Can you work these out from the model? Positions are in its coordinate system, mm. Round coordinates to 2 decimals unless told otherwise and drop trailing zeros. Loops run counter-clockwise (first coordinate to the right, second up) from the corner with the lowest first, then second, coordinate; pieces in that order, holes last.
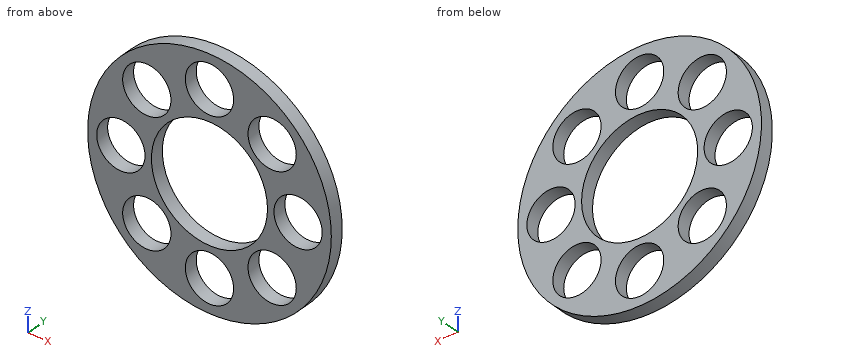
from build123d import *

# Parameters (mm, degrees)
F0_R     = 106
F0_R_2   = 50.5
F1_DEPTH = 6
F2_R     = 21
F3_DEPTH = 12
F4_DEPTH = 25


with BuildPart() as f1:
    # F0 (on Front) → F1 (new body, symmetric)
    with BuildSketch(Plane.XZ):
        Circle(F0_R)
        Circle(F0_R_2, mode=Mode.SUBTRACT)
    extrude(amount=F1_DEPTH, both=True)

    # F2 (on face) → F3 (join)
    with BuildSketch(Plane.XZ.offset(6)):
        with Locations((0, 77.0860096719)):
            Circle(F2_R)
        with Locations((54.5080401736, 54.5080401736)):
            Circle(F2_R)
        with Locations((77.0860096719, 0)):
            Circle(F2_R)
        with Locations((54.5080401736, -54.5080401736)):
            Circle(F2_R)
        with Locations((0, -77.0860096719)):
            Circle(F2_R)
        with Locations((-54.5080401736, -54.5080401736)):
            Circle(F2_R)
        with Locations((-77.0860096719, 0)):
            Circle(F2_R)
        with Locations((-54.5080401736, 54.5080401736)):
            Circle(F2_R)
    extrude(amount=F3_DEPTH)

    # F4 (cut, symmetric): faces of the model
    f4_faces = [f1.faces().sort_by_distance(p)[0] for p in [
        (-77.0860096719, -18, 0),
        (-54.5080401736, -18, 54.5080401736),
        (77.0860096719, -18, 0),
        (54.5080401736, -18, -54.5080401736),
        (0, -18, -77.0860096719),
        (-54.5080401736, -18, -54.5080401736),
        (0, -18, 77.0860096719),
        (54.5080401736, -18, 54.5080401736),
    ]]
    extrude(f4_faces, amount=F4_DEPTH, both=True, mode=Mode.SUBTRACT)


solid = f1.part
(1) If we section it at B-B, the plane x = 0: List the corners of the cut face in (y, z) for me, then the cut area to 3 significant figures.
Worked answers:
outline: (-6, -106) - (6, -106) - (6, -98.09) - (-6, -98.09) - close; (-6, -56.09) - (6, -56.09) - (6, -50.5) - (-6, -50.5) - close; (-6, 50.5) - (6, 50.5) - (6, 56.09) - (-6, 56.09) - close; (-6, 98.09) - (6, 98.09) - (6, 106) - (-6, 106) - close
area: 324 mm2
(2) If we section it at C-C, the plane y = 2: State how many separate pieces and enclosed holes the cut face has, then the cut area to 3 significant figures.
Worked answers:
separate pieces: 1
enclosed holes: 9
area: 16,200 mm2
(3) Will these pins go through, and if not, where does the flat tip stop? P1, Ø4, axis at y = 0, z = -7.5, coming from the +X side; P2, Ø25, axis at x = 0, z = 77.09, coming from the -Y side; P3, Ø5, axis at y = 1, z = 33.5, coming from the -X side; P4, Ø3, axis at x = 41, y = -0.5, coming from the -Z side.
Worked answers:
P1: stops at x = 105.86
P2: passes through
P3: stops at x = -101.37
P4: stops at z = -98.37
(4) If I drill on line 1 (Z direction, x = 0, y = 1.5); line 2 (X direction, y = 2.75, z = 1.5); line 3 (X direction, y = -3, z = -60), over which ranges is the centre line in solid material (lowest first)?
Worked answers:
line 1: z = -106 to -98.09, -56.09 to -50.5, 50.5 to 56.09, 98.09 to 106
line 2: x = -105.99 to -98.03, -56.14 to -50.48, 50.48 to 56.14, 98.03 to 105.99
line 3: x = -87.38 to -74.78, -34.24 to -12.21, 12.21 to 34.24, 74.78 to 87.38
(5) If we section it at D-D, the plane z = -90.5: List the corners of the cut face in (x, y) for me, then the cut area to 3 significant figures.
Worked answers:
outline: (-55.19, -6) - (-16.16, -6) - (-16.16, 6) - (-55.19, 6) - close; (16.16, -6) - (55.19, -6) - (55.19, 6) - (16.16, 6) - close
area: 937 mm2
(6) If we section it at A-A, the plane z = 0: List the corners of the cut face in (x, y) for me, then the cut area to 3 significant figures.
Worked answers:
outline: (-106, -6) - (-98.09, -6) - (-98.09, 6) - (-106, 6) - close; (-56.09, -6) - (-50.5, -6) - (-50.5, 6) - (-56.09, 6) - close; (50.5, -6) - (56.09, -6) - (56.09, 6) - (50.5, 6) - close; (98.09, -6) - (106, -6) - (106, 6) - (98.09, 6) - close
area: 324 mm2
